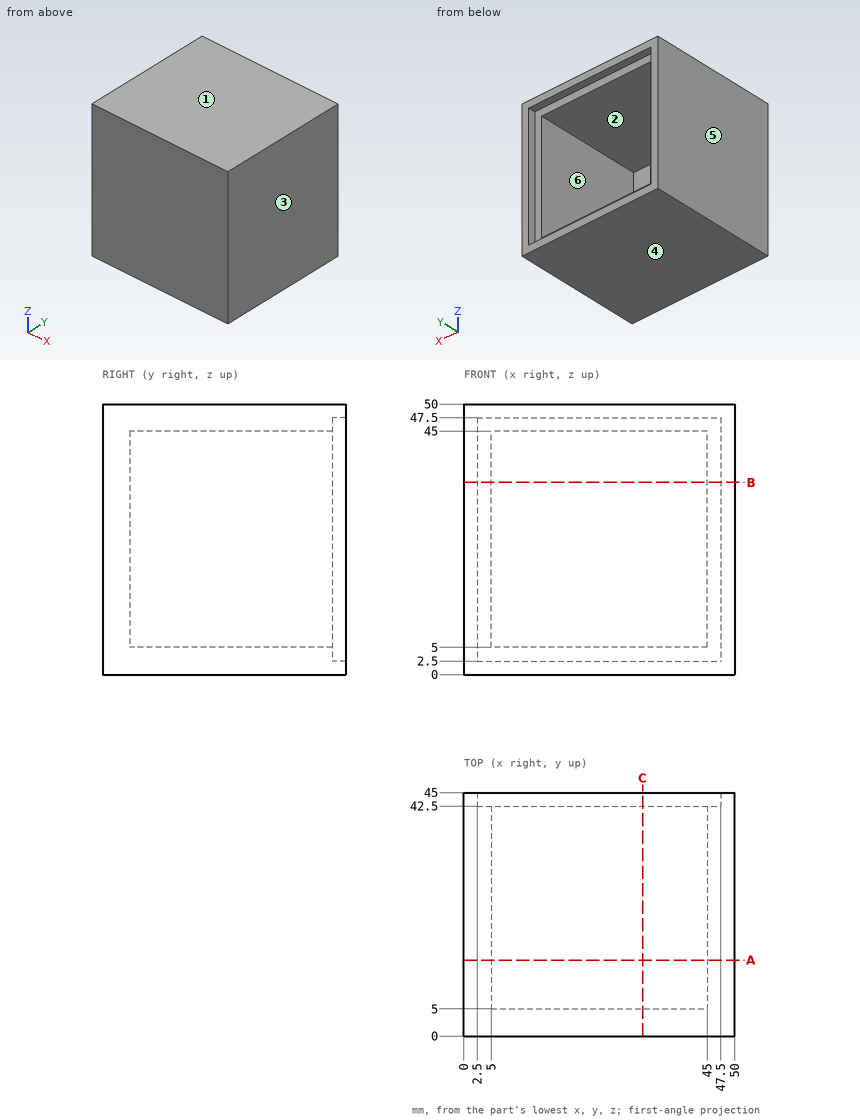
Answer from the drawing. Dimensions are ordinates in mm from the lowest x, y and z of the part. A direction names the side the tool comes from. Round coordinates to 2 decimals unless told otherwise and drop trailing zeros. Order: outer loops, then holes, each group sorted by start corner. A loop starts at its lowest first (then second) coordinate and runs counter-clockwise, first axis right, second up. Notation, with made-up numbers: (-40, 32.5) -> (-11, 32.5) arc R15 ccw to (-11, 55.5) -> close; hole circle Ø6 at (-19, 53). An arc over 180 degrees is marked (long way). Answer as CSV lines item,"result".
Q1. A cutting plane is placed at A-A on y = 14. Determine the outline of the cut face in (x, z), plus the area to 3 significant figures.
Computed values:
outline,"(0, 0) -> (50, 0) -> (50, 50) -> (0, 50) -> close; hole (5, 5) -> (45, 5) -> (45, 45) -> (5, 45) -> close"
area,"900 mm^2"
Q2. A cutting plane is placed at C-C on x = 33. Determine the outline of the cut face in (y, z).
Computed values:
outline,"(0, 0) -> (45, 0) -> (45, 2.5) -> (42.5, 2.5) -> (42.5, 5) -> (5, 5) -> (5, 45) -> (42.5, 45) -> (42.5, 47.5) -> (45, 47.5) -> (45, 50) -> (0, 50) -> close"
Q3. Given pin 1 (4 mm diameter, centred on x = 25, z = 32, fed in from +Y); pin 2 (5 mm diameter, centred on x = 26, z = 7, fed in from +Y), each flat-ended and moving along its own axis, determine where each tip first touches the part or whether it passes through.
Computed values:
pin 1,"stops at y = 5"
pin 2,"stops at y = 42.5"
Q4. Which of the six approach directions +Z, -Z, +X, -X, +Y, -Y give full straight-line access (tool end or side, diameter ignored) to the marked faces 5 and 6?
Computed values:
face 5,"+Z, -Z, -X, +Y, -Y"
face 6,"+Y"
Q5. A cutting plane is placed at B-B on z = 35.5. Determine the outline of the cut face in (x, y).
Computed values:
outline,"(0, 0) -> (50, 0) -> (50, 45) -> (47.5, 45) -> (47.5, 42.5) -> (45, 42.5) -> (45, 5) -> (5, 5) -> (5, 42.5) -> (2.5, 42.5) -> (2.5, 45) -> (0, 45) -> close"
Q6. For a pull along Z with two mould halves and no side action, classify the marked faces 1, 2, 3 and 4 as +Z half, -Z half, draft (parallel to the pull), parting line (faces both ways), or undercut.
Computed values:
face 1,"+Z half"
face 2,"undercut"
face 3,"draft"
face 4,"-Z half"
Q7. Consider line 1 (X direction, y = 37.5, z = 30); line 2 (Y direction, x = 41.5, z = 34). Determine where each line is inside the solid, lowest interval first. Write a range as from..to.
Computed values:
line 1,"x = 0..5, 45..50"
line 2,"y = 0..5"
